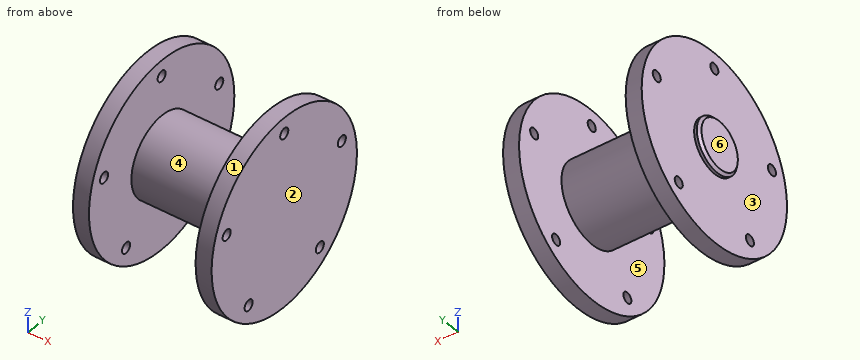
Autodesk Inventor part; units mm, degrees
ref_plane "YZ Plane" through (0, 0, 0) normal (1, 0, 0) x (0, 1, 0)
ref_plane "XZ Plane" through (0, 0, 0) normal (0, 1, 0) x (-1, 0, 0)
ref_plane "XY Plane" through (0, 0, 0) normal (0, 0, 1) x (1, 0, 0)
sketch "スケッチ1" plane through (0, 0, 0) normal (1, 0, 0) x (0, 1, 0)
  circle A0 centre (0, 0) radius 36
  dimension "d0" = 72
extrude "押し出し1" add sketch "スケッチ1" along normal blind 6
sketch "スケッチ2" plane through (6, 0, 0) normal (1, 0, 0) x (0, 0, -1)
  circle A0 centre (0, 0) radius 15
  dimension "d3" = 30
extrude "押し出し2" add sketch "スケッチ2" along normal blind 40
sketch "スケッチ3" plane through (46, 0, 0) normal (1, 0, 0) x (0, 0, -1)
  circle A0 centre (0, 0) radius 36
  dimension "d6" = 72
extrude "押し出し3" add sketch "スケッチ3" along normal blind 6
sketch "スケッチ4" plane through (0, 0, 0) normal (-1, 0, 0) x (0, 0, 1)
  circle A0 centre (30, 0) radius 2
  circle A1 centre (9.2705, 28.5317) radius 2
  circle A2 centre (-24.2705, 17.6336) radius 2
  circle A3 centre (-24.2705, -17.6336) radius 2
  circle A4 centre (9.2705, -28.5317) radius 2
  circle A5 centre (0, 0) radius 10
  dimension "d9" = 30
  dimension "d10" = 4
  dimension "d13" = 360
  dimension "d17" = 20
extrude "押し出し4" cut sketch "スケッチ4" against normal blind 6 contours A0 | A1 | A2 | A3 | A4
extrude "押し出し5" add sketch "スケッチ4" along normal blind 2 contours A5
chamfer "面取り1" distance 1 angle 45 1 edges at (-2, 0, -10)
sketch "スケッチ6" plane through (52, 0, 0) normal (1, 0, 0) x (0, 0, -1)
  circle A0 centre (24.2705, 17.6336) radius 2
  circle A1 centre (24.2705, 17.6336) radius 2
  circle A2 centre (-9.2705, 28.5317) radius 2
  circle A3 centre (-9.2705, 28.5317) radius 2
  circle A4 centre (-30, 0) radius 2
  circle A5 centre (24.2705, -17.6336) radius 2
  circle A6 centre (24.2705, -17.6336) radius 2
  circle A7 centre (-9.2705, -28.5317) radius 2
  circle A8 centre (-9.2705, -28.5317) radius 2
  point P0 (0, 0)
extrude "押し出し6" cut sketch "スケッチ6" against normal blind 6
properties part number "tool_1" material "アルミニウム 6061"
Source: CAD feature listing. Evaluate the final solid. Frame: model axes, mm. Face numbers are marked on the shaded views. A direction names the side the tool comes from. Coordinates: 2 decimals unless noted, no trailing zeros. Order: outer loops, then holes, each group sorted by start corner. A loop starts at its lowest first (then second) coordinate and runs counter-clockwise, first axis right, second up. Notation, with made-up numbers: (9.25, -31) - (31.25, -31) arc R7 cw to (31.25, -19) - close; hole circle Ø8 at (36.25, -29.5). An arc over 180 degrees is marked (long way). One line per item, written item: value.
1) Contact query for flat-ended pins moving along their axis: pin 1 (10 mm diameter, centred on x = 17.5, y = -12.5, fed in from -Z); pin 2 (5 mm diameter, centred on x = 7.5, y = 3.5, fed in from -Z); pin 3 (6 mm diameter, centred on x = 20, y = 0, fed in from +Z). Output: stop coordinate, or through.
Computed values:
pin 1: stops at z = -12.99
pin 2: stops at z = -35.97
pin 3: stops at z = 15
2) Reachability of the marked faces 5 and 6 from +Z, -Z, +X, -X, +Y, -Y: full face, straight path, thin tool, end or side. Return the list, or none.
Computed values:
face 5: none
face 6: +Z, -Z, -X, +Y, -Y
3) Ray query, line 1 (X direction, y = -4.5, z = 30); line 2 (X direction, y = -10, z = -4); line 3 (Y direction, x = 47.65, z = 30). Return the intervals inside material, ascending. Write a range as [from, to].
Computed values:
line 1: x = [0, 6], [46, 52]
line 2: x = [0, 52]
line 3: y = [-19.9, -2], [2, 19.9]
4) Cut plane B-B on z = -25. Output: boundary loops of the cut face in (x, y).
Computed values:
outline: (0, -25.9) - (6, -25.9) - (6, -19.5) - (0, -19.5) - close; (0, -15.77) - (6, -15.77) - (6, 15.77) - (0, 15.77) - close; (0, 19.5) - (6, 19.5) - (6, 25.9) - (0, 25.9) - close; (46, -25.9) - (52, -25.9) - (52, -19.5) - (46, -19.5) - close; (46, -15.77) - (52, -15.77) - (52, 15.77) - (46, 15.77) - close; (46, 19.5) - (52, 19.5) - (52, 25.9) - (46, 25.9) - close
5) Cut plane A-A on y = 0. Output: boundary loops of the cut face in (x, z).
Computed values:
outline: (-2, -9) - (-1, -10) - (0, -10) - (0, -36) - (6, -36) - (6, -15) - (46, -15) - (46, -36) - (52, -36) - (52, 28) - (46, 28) - (46, 15) - (6, 15) - (6, 28) - (0, 28) - (0, 10) - (-1, 10) - (-2, 9) - close; (0, 32) - (6, 32) - (6, 36) - (0, 36) - close; (46, 32) - (52, 32) - (52, 36) - (46, 36) - close
6) Cut plane C-C on z = 0. Output: boundary loops of the cut face in (x, y), plus the area to 3 significant figures.
Computed values:
outline: (-2, -9) - (-1, -10) - (0, -10) - (0, -36) - (6, -36) - (6, -15) - (46, -15) - (46, -36) - (52, -36) - (52, 36) - (46, 36) - (46, 15) - (6, 15) - (6, 36) - (0, 36) - (0, 10) - (-1, 10) - (-2, 9) - close
area: 2,100 mm^2
7) Cut plane D-D on z = 30. Output: boundary loops of the cut face in (x, y), plus the area to 3 significant figures.
Computed values:
outline: (0, -19.9) - (6, -19.9) - (6, -2) - (0, -2) - close; (0, 2) - (6, 2) - (6, 19.9) - (0, 19.9) - close; (46, -19.9) - (52, -19.9) - (52, -2) - (46, -2) - close; (46, 2) - (52, 2) - (52, 19.9) - (46, 19.9) - close
area: 430 mm^2
8) Mould query, pull axis X, two halves, no side actions, for the marked faces 1, 2, 3 and 4. Classes: released by +X, released by -X, zero draft, split by the parting line, or undercut.
Computed values:
face 1: zero draft
face 2: released by +X
face 3: released by -X
face 4: undercut
